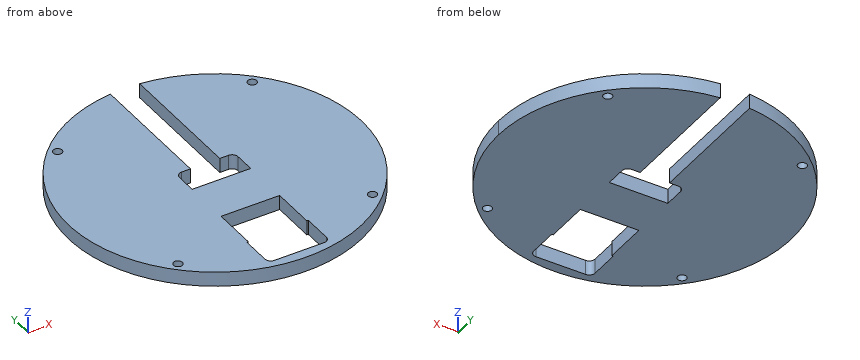
```python
from build123d import *

# Parameters (mm, degrees)
SKETCH_1_R      = 1.5
EXTRUDE_1_DEPTH = 5


with BuildPart() as part:
    # 草图1 → 凸台-拉伸1 (new body)
    with BuildSketch(Plane.XY):
        with BuildLine():
            Line((-5, 5.5), (-5, 49.749371855))
            ThreePointArc((-5, 49.749371855), (-33.541019662, -37.080992435), (50, 0))
            ThreePointArc((50, 0), (37.080992435, 33.541019662), (5, 49.749371855))
            Line((5, 49.749371855), (5, 5.5))
            Line((5, 5.5), (8, 5.5))
            ThreePointArc((8, 5.5), (9.414213562, 4.914213562), (10, 3.5))
            Line((10, 3.5), (10, -3.5))
            Line((10, -3.5), (-10, -3.5))
            Line((-10, -3.5), (-10, 3.5))
            ThreePointArc((-10, 3.5), (-9.414213562, 4.914213562), (-8, 5.5))
            Line((-8, 5.5), (-5, 5.5))
        make_face()
        with Locations((-33.234018716, -33.234018716)):
            Circle(SKETCH_1_R, mode=Mode.SUBTRACT)
        with BuildLine():
            Line((-10.5, -34.5), (-10, -34.5))
            Line((-10, -34.5), (-10, -19.5))
            Line((-10, -19.5), (10, -19.5))
            Line((10, -19.5), (10, -34.5))
            Line((10, -34.5), (10.5, -34.5))
            Line((10.5, -34.5), (10.5, -44.5))
            ThreePointArc((10.5, -44.5), (9.914213562, -45.914213562), (8.5, -46.5))
            Line((8.5, -46.5), (-8.5, -46.5))
            ThreePointArc((-8.5, -46.5), (-9.914213562, -45.914213562), (-10.5, -44.5))
            Line((-10.5, -44.5), (-10.5, -34.5))
        make_face(mode=Mode.SUBTRACT)
        with Locations((33.234018716, -33.234018716)):
            Circle(SKETCH_1_R, mode=Mode.SUBTRACT)
        with Locations((-33.234018716, 33.234018716)):
            Circle(SKETCH_1_R, mode=Mode.SUBTRACT)
        with Locations((33.234018716, 33.234018716)):
            Circle(SKETCH_1_R, mode=Mode.SUBTRACT)
    extrude(amount=EXTRUDE_1_DEPTH)


solid = part.part
```
CAD build for the part. Positions are in the model's coordinates, mm. Round coordinates to 2 decimals unless told otherwise and drop trailing zeros. Loops run counter-clockwise (first coordinate to the right, second up) from the corner with the lowest first, then second, coordinate; pieces in that order, holes last. Notation, with made-up numbers: M 36,2.25 L 55,2.25 A16 ccw 55,6.25 Z; hole C -9.5,53.25 d9. An arc over 180 degrees is marked long. Use a Markdown table: item, result. Add a question column.
(1) Drill centre lines: line 1 (X direction, y = 32.5, z = 0.45); line 2 (Y direction, x = -33.5, z = 4.2); line 3 (X direction, y = -32.5, z = 0.35). Where is each one in solid material? Low to high.
(2) Cut at C-C (z = 1.7). Give the cut face in (x, y).
(3) Cut at A-A (x = 0). Give the cut face in (y, z), and give its area (3 significant figures).
(4) Cut at B-B (y = -27). Give the cut face in (x, z), and give its area (3 significant figures).
(5) Flat gauge pins, fed straight in: pin 1 (1 mm diameter, centred on y = -14, z = 4, fed in from +X); pin 2 (1 mm diameter, centred on x = -11.5, y = -30.5, fed in from -Z); pin 3 (2.5 mm diameter, centred on x = 2, z = 3.5, fed in from -Y); pin 4 (1.5 mm diameter, centred on y = -37.5, z = 1.5, fed in from +X). Where does each tip first touch, or does it go through?
Geometry says:
| question | item | result |
|---|---|---|
| 1 | line 1 | x = -38 to -34.54, -31.93 to -5, 5 to 31.93, 34.54 to 38 |
| 1 | line 2 | y = -37.12 to -34.71, -31.76 to 31.76, 34.71 to 37.12 |
| 1 | line 3 | x = -38 to -34.54, -31.93 to -10, 10 to 31.93, 34.54 to 38 |
| 2 | outline | M -10,-3.5 L -10,3.5 A2 cw -8,5.5 L -5,5.5 L -5,49.75 A50 ccw long 5,49.75 L 5,5.5 L 8,5.5 A2 cw 10,3.5 L 10,-3.5 Z; hole C -33.23,-33.23 d3; hole C -33.23,33.23 d3; hole M -10.5,-44.5 A2 ccw -8.5,-46.5 L 8.5,-46.5 A2 ccw 10.5,-44.5 L 10.5,-34.5 L 10,-34.5 L 10,-19.5 L -10,-19.5 L -10,-34.5 L -10.5,-34.5 Z; hole C 33.23,-33.23 d3; hole C 33.23,33.23 d3 |
| 3 | outline | M -50,0 L -46.5,0 L -46.5,5 L -50,5 Z; M -19.5,0 L -3.5,0 L -3.5,5 L -19.5,5 Z |
| 3 | area | 97.5 mm² |
| 4 | outline | M -42.08,0 L -10,0 L -10,5 L -42.08,5 Z; M 10,0 L 42.08,0 L 42.08,5 L 10,5 Z |
| 4 | area | 321 mm² |
| 5 | pin 1 | stops at x = 48.14 |
| 5 | pin 2 | stops at z = 0 |
| 5 | pin 3 | stops at y = -49.99 |
| 5 | pin 4 | stops at x = 33.9 |
